For this review, take the finished solid that the model builds, in its own axes (mm). A direction names the side the tool comes from. Give positions to 0.01 mm unless a question says otherwise; leave off trailing zeros. Loops run counter-clockwise (first coordinate to the right, second up) from the corner with the lowest first, then second, coordinate; pieces in that order, holes last. Notation, with made-up numbers: (-0.75, 84.5) - (8.25, 84.5) arc R5 cw to (8.25, 92.5) - close; hole circle Ø1 at (-37, 70.5). An arc over 180 degrees is marked (long way). Use CSV: the item, a comma, the result in double quotes. Start each with the question number.
1. Take a section at A-A on y = 4. Give the boundary of the cut face in (x, z).
2. For pin 1 (1 mm diameter, centred on x = 1.5, z = -1.5, fed in from -Y); pin 2 (1.5 mm diameter, centred on y = 19.5, z = -1, fed in from +X); pin 3 (2 mm diameter, centred on y = 49.5, z = -1.5, fed in from -X); pin 4 (3 mm diameter, centred on y = 14.5, z = 1, fed in from +X), all flat-tipped, find the tip position at first contact; note any pin that passes through.
3. Take a section at D-D on y = 39.5. Give the boundary of the cut face in (x, z), plus the area to 3 significant figures.
4. Take a section at C-C on z = -0.6. Give the boundary of the cut face in (x, y), plus the area to 3 significant figures.
5. Wall thickness on line 1 (X direction, y = 31.5, z = -0.65); line 2 (Z direction, x = 1.8, y = 47); line 3 (Z direction, x = -1.3, y = 3.5): over which ranges is each line inside the solid? List them lowest first.
6. For faces 1 (the flat face through (2.175, 28.535, -1.233)), 2 (the flat face through (1.328, 51.35, -2.295)), 3 (the flat face through (1.328, 6.35, -2.295)), list the 3-axis set-ups (+Z, -Z, +X, -X, +Y, -Y) from which the entire face can be reached by the end or side of a thin tool; tool diameter is ignored.
7. Take a section at B-B on x = -0.95. Give the boundary of the cut face in (y, z).
```python
from build123d import *

# Parameters (mm, degrees)
BOSS_EXTRUDE1_DEPTH = 57.699999944
CUT_EXTRUDE1_DEPTH  = 6.35


with BuildPart() as part:
    # Sketch1 → Boss-Extrude1 (new body)
    with BuildSketch(Plane(origin=(0, 0, 0), x_dir=(1, 0, 0), z_dir=(0, 1, 0))):
        Polygon((2.886751346, 0), (1.443375673, 2.5), (-1.443375673, 2.5), (-2.886751346, 0), (-1.443375673, -2.5), (1.443375673, -2.5), align=None)
    extrude(amount=BOSS_EXTRUDE1_DEPTH)

    # Sketch2 → Cut-Extrude1 (cut)
    with BuildSketch(Plane(origin=(0, 0, 0), x_dir=(-1, 0, 0), z_dir=(0, -1, 0))):
        with BuildLine():
            Line((-2.16506344, -1.25000012), (-1.443375673, -2.5))
            Line((-1.443375673, -2.5), (0, -2.5))
            ThreePointArc((0, -2.5), (-1.24999994, -2.165063544), (-2.16506344, -1.25000012))
        make_face()
        with BuildLine():
            Line((0, -2.5), (1.443375673, -2.5))
            Line((1.443375673, -2.5), (2.165063522, -1.249999979))
            ThreePointArc((2.165063522, -1.249999979), (1.250000011, -2.165063503), (0, -2.5))
        make_face()
        with BuildLine():
            Line((2.165063522, -1.249999979), (2.886751346, 0))
            Line((2.886751346, 0), (2.165063508, 1.250000002))
            ThreePointArc((2.165063508, 1.250000002), (2.414814565, 0.647047614), (2.5, 0))
            ThreePointArc((2.5, 0), (2.414814569, -0.647047601), (2.165063522, -1.249999979))
        make_face()
        with BuildLine():
            Line((2.165063508, 1.250000002), (1.443375673, 2.5))
            Line((1.443375673, 2.5), (0, 2.5))
            ThreePointArc((0, 2.5), (1.249999999, 2.16506351), (2.165063508, 1.250000002))
        make_face()
        with BuildLine():
            Line((-2.165063434, 1.25000013), (-2.886751346, 0))
            Line((-2.886751346, 0), (-2.16506344, -1.25000012))
            ThreePointArc((-2.16506344, -1.25000012), (-2.5, 6e-09), (-2.165063434, 1.25000013))
        make_face()
        with BuildLine():
            Line((0, 2.5), (-1.443375673, 2.5))
            Line((-1.443375673, 2.5), (-2.165063434, 1.25000013))
            ThreePointArc((-2.165063434, 1.25000013), (-1.249999935, 2.165063547), (0, 2.5))
        make_face()
    cut_extrude1 = extrude(amount=-CUT_EXTRUDE1_DEPTH, mode=Mode.SUBTRACT)

    # Mirror1: Cut-Extrude1 across plane
    add(cut_extrude1.mirror(Plane(origin=(0, 28.849999972, 0), x_dir=(0, 0, 1), z_dir=(0, -1, 0))), mode=Mode.SUBTRACT)


solid = part.part
```
Check result:
1,outline,"circle Ø5 at (0, 0)"
2,pin 1,"stops at y = 0"
2,pin 2,"stops at x = 2.74"
2,pin 3,"stops at x = -2.6"
2,pin 4,"stops at x = 2.89"
3,outline,"(-2.89, 0) - (-1.44, -2.5) - (1.44, -2.5) - (2.89, 0) - (1.44, 2.5) - (-1.44, 2.5) - close"
3,area,"21.7 mm²"
4,outline,"(-2.54, 6.35) - (-2.43, 6.35) - (-2.43, 0) - (2.43, 0) - (2.43, 6.35) - (2.54, 6.35) - (2.54, 51.35) - (2.43, 51.35) - (2.43, 57.7) - (-2.43, 57.7) - (-2.43, 51.35) - (-2.54, 51.35) - close"
4,area,"290 mm²"
5,line 1,"x = -2.51 to 2.51"
5,line 2,"z = -1.88 to 1.88"
5,line 3,"z = -2.14 to 2.14"
6,face 1,"-Z, +X, +Y, -Y"
6,face 2,"-Z, +X, +Y"
6,face 3,"-Z, +X, -Y"
7,outline,"(0, -2.31) - (6.35, -2.31) - (6.35, -2.5) - (51.35, -2.5) - (51.35, -2.31) - (57.7, -2.31) - (57.7, 2.31) - (51.35, 2.31) - (51.35, 2.5) - (6.35, 2.5) - (6.35, 2.31) - (0, 2.31) - close"
